```python
from build123d import *

# Parameters (mm, degrees)
SKETCH1_W           = 8.08
SKETCH1_H           = 5.65
BOSS_EXTRUDE1_DEPTH = 2.72
CUT_EXTRUDE1_DEPTH  = 4


with BuildPart() as part:
    # Sketch1 → Boss-Extrude1 (new body)
    with BuildSketch(Plane.XY):
        with Locations((4.04, 2.825)):
            Rectangle(SKETCH1_W, SKETCH1_H)
    extrude(amount=BOSS_EXTRUDE1_DEPTH)

    # Sketch2 → Cut-Extrude1 (cut)
    with BuildSketch(Plane.XZ):
        Polygon((0.54, 2.3), (7.54, 2.3), (6.425, 0.42), (1.655, 0.42), align=None)
    extrude(amount=-CUT_EXTRUDE1_DEPTH, mode=Mode.SUBTRACT)


solid = part.part
```
Check sheet for the modelled part. Datum: model origin and axes. Units: mm. A direction names the side the tool comes from. Round coordinates to 2 decimals unless told otherwise and drop trailing zeros. Order: outer loops, then holes, each group sorted by start corner. A loop starts at its lowest first (then second) coordinate and runs counter-clockwise, first axis right, second up. Notation, with made-up numbers: M -31,3 L -22,3 A5 cw -22,11 Z; hole C -19,59.5 d3. An arc over 180 degrees is marked long. Answer in a Markdown table with one row per item.
(1) Set-up check for faces 1 (the flat face through (6.99, 1.97, 1.37)), 2 (the flat face through (4, 3, 2.72)): record each of +Z, -Z, +X, -X, +Y, -Y from which the full face is reachable in a straight line by a thin tool's end or side.
Findings:
| item | result |
|---|---|
| face 1 | -Y |
| face 2 | +Z, +X, -X, +Y, -Y |
(2) Gauge pin test, flat end, axial feed: pin 1 (0.9 mm diameter, centred on x = 3.5, z = 1, fed in from -Y). Record the tip position at first contact, or that the pin passes through.
Findings:
| item | result |
|---|---|
| pin 1 | stops at y = 4 |
(3) Section check A-A on y = 3.9. Record the boundary of the cut face in (x, z) (3 decimals), plus the area to 3 significant figures.
Findings:
| item | result |
|---|---|
| outline | M 0,0 L 8.08,0 L 8.08,2.72 L 0,2.72 Z; hole M 0.54,2.3 L 1.655,0.42 L 6.425,0.42 L 7.54,2.3 Z |
| area | 10.9 mm^2 |
(4) Section check B-B on x = 2.75. Record the boundary of the cut face in (y, z).
Findings:
| item | result |
|---|---|
| outline | M 0,0 L 5.65,0 L 5.65,2.72 L 0,2.72 L 0,2.3 L 4,2.3 L 4,0.42 L 0,0.42 Z |
(5) Section check C-C on z = 0.6. Record the boundary of the cut face in (x, y), plus the area to 3 significant figures.
Findings:
| item | result |
|---|---|
| outline | M 0,0 L 1.55,0 L 1.55,4 L 6.53,4 L 6.53,0 L 8.08,0 L 8.08,5.65 L 0,5.65 Z |
| area | 25.7 mm^2 |
(6) Material ranges on line 1 along Z through (x, y) = (5.75, 1.9); line 2 along Y through (x, z) = (6.5, 1.5); line 3 along Z through (x, y) = (1.25, 2.35), recorded low to high. Write a range as from..to.
Findings:
| item | result |
|---|---|
| line 1 | z = 0..0.42, 2.3..2.72 |
| line 2 | y = 4..5.65 |
| line 3 | z = 0..1.1, 2.3..2.72 |
(7) Draft check along Z on faces 3 (the flat face through (4, 5.65, 1)), 4 (the flat face through (4, 3, 0)), 5 (the flat face through (1.105, 1.972, 1.347)), 6 (the flat face through (4, 2, 2.3)). Enter one of: +Z half, -Z half, draft (parallel to the pull), parting line (faces both ways), or undercut.
Findings:
| item | result |
|---|---|
| face 3 | draft |
| face 4 | -Z half |
| face 5 | undercut |
| face 6 | undercut |
